The listing builds one solid part. Answer for the finished solid, in the listing's coordinates (mm). Round coordinates to 2 decimals unless told otherwise and drop trailing zeros. Write each loop counter-clockwise with the first axis right and the second up, starting at its lowest first coordinate (ties: lowest second). Pieces come first, ordered by that corner, then holes.
(1) Find the intervals of material crossed by probe 1 along X at (y, z) = (0.8, -5); probe 2 along Z at (x, y) = (32.5, 0.3); probe 3 along Z at (x, y) = (-12, 0.8), in increasing order.
(2) A cutting plane is placed at D-D, the plane z = 1.5. Give the vertices of the cut face in (x, y), and give its area (3 significant figures).
(3) A cutting plane is placed at C-C, the plane x = -9. Give the vertices of the cut face in (y, z), and give its area (3 significant figures).
(4) This flat-tipped pin is pushed along its axis until it touches: pin 1 Ø10 at (x, z) = (-44, -3) entering from -Y. Where does it stop, or does it pass through?
(5) A cutting plane is placed at A-A, the plane z = -4. Give the vertices of the cut face in (x, y).
(6) A cutting plane is placed at B-B, the plane y = 0.6. Give the vertices of the cut face in (x, z), and give its area (3 significant figures).
from build123d import *

# Parameters (mm, degrees)
F0_W     = 27
F0_H     = 3
F0_W_2   = 8
F0_H_2   = 3.1
F0_W_3   = 8.8
F0_H_3   = 11.3
F1_DEPTH = 1


with BuildPart() as f1:
    # F0 (on Front) → F1 (new body)
    with BuildSketch(Plane.XZ):
        with BuildLine():
            Line((64, 15), (-64, 15))
            ThreePointArc((-64, 15), (-66.12132, 14.12132), (-67, 12))
            Line((-67, 12), (-67, -12))
            ThreePointArc((-67, -12), (-66.12132, -14.12132), (-64, -15))
            Line((-64, -15), (64, -15))
            ThreePointArc((64, -15), (66.12132, -14.12132), (67, -12))
            Line((67, -12), (67, 12))
            ThreePointArc((67, 12), (66.12132, 14.12132), (64, 15))
        make_face()
        with Locations((-5.3, -8.1)):
            Rectangle(F0_W, F0_H, mode=Mode.SUBTRACT)
        with Locations((17.7, -3.75)):
            Rectangle(F0_W_2, F0_H_2, mode=Mode.SUBTRACT)
        with Locations((33.1, 0.35)):
            Rectangle(F0_W_3, F0_H_3, mode=Mode.SUBTRACT)
    extrude(amount=-F1_DEPTH)


solid = f1.part
Solutions:
1. probe 1: x = -67 to 13.7, 21.7 to 28.7, 37.5 to 67
1. probe 2: z = -15 to -5.3, 6 to 15
1. probe 3: z = -15 to -9.6, -6.6 to 15
2. outline: (-67, 0) - (28.7, 0) - (28.7, 1) - (-67, 1) - close; (37.5, 0) - (67, 0) - (67, 1) - (37.5, 1) - close
2. area: 125 mm2
3. outline: (0, -15) - (1, -15) - (1, -9.6) - (0, -9.6) - close; (0, -6.6) - (1, -6.6) - (1, 15) - (0, 15) - close
3. area: 27.0 mm2
4. pin 1: stops at y = 0
5. outline: (-67, 0) - (13.7, 0) - (13.7, 1) - (-67, 1) - close; (21.7, 0) - (28.7, 0) - (28.7, 1) - (21.7, 1) - close; (37.5, 0) - (67, 0) - (67, 1) - (37.5, 1) - close
6. outline: (-67, -12) arc R3 ccw to (-64, -15) - (64, -15) arc R3 ccw to (67, -12) - (67, 12) arc R3 ccw to (64, 15) - (-64, 15) arc R3 ccw to (-67, 12) - close; hole (-18.8, -9.6) - (8.2, -9.6) - (8.2, -6.6) - (-18.8, -6.6) - close; hole (13.7, -5.3) - (21.7, -5.3) - (21.7, -2.2) - (13.7, -2.2) - close; hole (28.7, -5.3) - (37.5, -5.3) - (37.5, 6) - (28.7, 6) - close
6. area: 3,810 mm2
